Build history of the part. All positions in model axes, mm. Face numbers are marked on the shaded views. A direction names the side the tool comes from. Give positions to 0.01 mm unless a question says otherwise; leave off trailing zeros. Order: outer loops, then holes, each group sorted by start corner. A loop starts at its lowest first (then second) coordinate and runs counter-clockwise, first axis right, second up. Notation, with made-up numbers: M 11,66 L 19,66 A22 cw 19,88 Z; hole C -38.5,40 d11. An arc over 180 degrees is marked long. Answer as CSV lines item,"result".
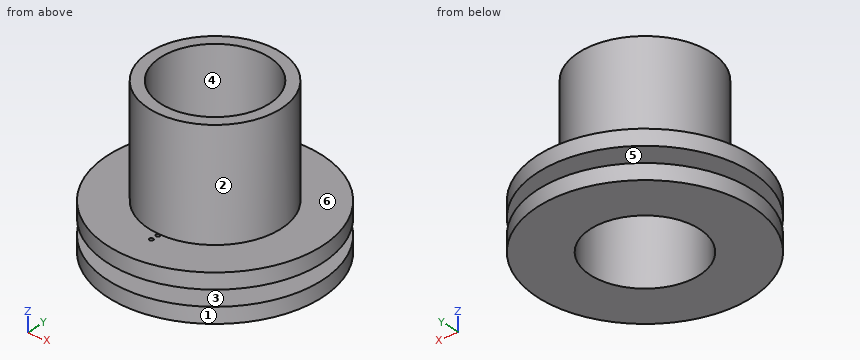
from build123d import *

# Parameters (mm, degrees)
SKETCH1_R           = 13.75
BOSS_EXTRUDE1_DEPTH = 2
SKETCH2_R           = 8.5
BOSS_EXTRUDE2_DEPTH = 6
BOSS_EXTRUDE3_START = 4
SKETCH3_R           = 13.75
BOSS_EXTRUDE3_DEPTH = 2
SKETCH5_R           = 7
CUT_EXTRUDE2_DEPTH  = 21.350061425
BOSS_EXTRUDE4_START = 6
SKETCH6_R           = 8.5
SKETCH6_R_2         = 7
BOSS_EXTRUDE4_DEPTH = 14
CUT_EXTRUDE3_START  = 4
SKETCH9_R           = 0.25
CUT_EXTRUDE3_DEPTH  = 24.894892006


with BuildPart() as part:
    # Sketch1 → Boss-Extrude1 (new body)
    with BuildSketch(Plane.XY):
        Circle(SKETCH1_R)
    extrude(amount=BOSS_EXTRUDE1_DEPTH)

    # Sketch2 → Boss-Extrude2 (add)
    with BuildSketch(Plane.XY):
        Circle(SKETCH2_R)
    extrude(amount=BOSS_EXTRUDE2_DEPTH)

    # Sketch3 → Boss-Extrude3 (add)
    with BuildSketch(Plane.XY.offset(BOSS_EXTRUDE3_START)):
        Circle(SKETCH3_R)
    extrude(amount=BOSS_EXTRUDE3_DEPTH)

    # Sketch5 → Cut-Extrude2 (cut, through all)
    with BuildSketch(Plane.XY):
        Circle(SKETCH5_R)
    extrude(amount=CUT_EXTRUDE2_DEPTH, mode=Mode.SUBTRACT)

    # Sketch6 → Boss-Extrude4 (add)
    with BuildSketch(Plane.XY.offset(BOSS_EXTRUDE4_START)):
        Circle(SKETCH6_R)
        Circle(SKETCH6_R_2, mode=Mode.SUBTRACT)
    extrude(amount=BOSS_EXTRUDE4_DEPTH)

    # Sketch9 → Cut-Extrude3 (cut, through all)
    with BuildSketch(Plane.XY.offset(CUT_EXTRUDE3_START)):
        with Locations((0, 9.75)):
            Circle(SKETCH9_R)
        with Locations((0, -9.75)):
            Circle(SKETCH9_R)
        with Locations(Location((0, 8.75, 0), (0, 0, 270.001597254))):
            Circle(SKETCH9_R)
        with Locations(Location((0, -8.75, 0), (0, 0, 90.001597254))):
            Circle(SKETCH9_R)
    extrude(amount=CUT_EXTRUDE3_DEPTH, mode=Mode.SUBTRACT)


solid = part.part
Item 1: Band-saw the part on C-C (x = 9). Give the cut face in (y, z), and give its area (3 significant figures).
Geometry says:
outline,"M -10.4,0 L 10.4,0 L 10.4,2 L -10.4,2 Z; M -10.4,4 L 10.4,4 L 10.4,6 L -10.4,6 Z"
area,"83.2 mm2"
Item 2: Probe line 1 along Y through (x, z) = (0, 4.8); line 2 along Z through (x, y) = (-10.25, -5.5); line 3 along X through (y, z) = (5.25, 13). List the from-to ranges inside material, lowest first. Write a range as from..to.
Geometry says:
line 1,"y = -13.75..-10, -9.5..-9, -8.5..-7, 7..8.5, 9..9.5, 10..13.75"
line 2,"z = 0..2, 4..6"
line 3,"x = -6.68..-4.63, 4.63..6.68"
Item 3: Band-saw the part on A-A (y = 0). Give the cut face in (x, z), and give its area (3 significant figures).
Geometry says:
outline,"M -13.75,0 L -7,0 L -7,20 L -8.5,20 L -8.5,6 L -13.75,6 L -13.75,4 L -8.5,4 L -8.5,2 L -13.75,2 Z; M 7,0 L 13.75,0 L 13.75,2 L 8.5,2 L 8.5,4 L 13.75,4 L 13.75,6 L 8.5,6 L 8.5,20 L 7,20 Z"
area,"102 mm2"
Item 4: Band-saw the part on B-B (x = -12). Give the cut face in (y, z).
Geometry says:
outline,"M -6.71,0 L 6.71,0 L 6.71,2 L -6.71,2 Z; M -6.71,4 L 6.71,4 L 6.71,6 L -6.71,6 Z"
Item 5: Band-saw the part on D-D (y = 4). Give the cut face in (x, z), and give its area (3 significant figures).
Geometry says:
outline,"M -13.16,0 L -5.74,0 L -5.74,20 L -7.5,20 L -7.5,6 L -13.16,6 L -13.16,4 L -7.5,4 L -7.5,2 L -13.16,2 Z; M 5.74,0 L 13.16,0 L 13.16,2 L 7.5,2 L 7.5,4 L 13.16,4 L 13.16,6 L 7.5,6 L 7.5,20 L 5.74,20 Z"
area,"115 mm2"
Item 6: Pull direction Z, two halves, no side cores. Call the marked faces 4, 5 and 6: released by +Z, released by -Z, zero draft, split by the parting line, or undercut.
Geometry says:
face 4,"zero draft"
face 5,"undercut"
face 6,"released by +Z"
Item 7: 3-axis set-ups, long thin cutter, end or side, ignore diameter. For the marked faces 1, 2 and 3: which of +Z, -Z, +X, -X, +Y, -Y reach the whole face in a straight line?
Geometry says:
face 1,"+Z, -Z"
face 2,"+Z"
face 3,"none"
Item 8: Drop flat-ended pins along their axis: pin 1 (4 mm diameter, centred on x = 0, z = 12, fed in from -Y); pin 2 (8 mm diameter, centred on y = -2, z = 7.5, fed in from -X); pin 3 (5 mm diameter, centred on y = -6, z = 11.5, fed in from -X); pin 4 (8.5 mm diameter, centred on x = 0, y = 0, fed in from +Z). Give the stop position or say it passes through.
Geometry says:
pin 1,"stops at y = -8.5"
pin 2,"stops at x = -13.75"
pin 3,"stops at x = -7.75"
pin 4,"passes through"
